The model under review builds one solid part; all positions refer to its coordinate system, in mm. Coordinates: 2 decimals unless noted, no trailing zeros. Loops run counter-clockwise (first coordinate to the right, second up) from the corner with the lowest first, then second, coordinate; pieces in that order, holes last. Notation, with made-up numbers: (-30, 83) - (27, 83) arc R15 ccw to (27, 97) - close; hole circle Ø8 at (-5.75, 38). An arc over 180 degrees is marked (long way). Answer in a Markdown table with one row per item. Add a question column.
(1) For P1, Ø5.5, axis at x = 137.85, z = -83.65, coming from the +Y side; P2, Ø2.5, axis at x = -47.65, z = 80.65, coming from the -Y side; P3, Ø1.5, axis at x = -39, y = 7, coming from the +Z side (3 decimals); P4, Ø5, axis at x = 54.5, z = 102, coming from the +Y side, all flat-tipped, find the tip position at first contact; note any pin that passes through.
(2) We need section B-B on x = 194. Write out the cut boundary in (y, z) (3 decimals), plus the area to 3 significant figures.
(3) For line 1 along X through (y, z) = (5, -0.5); line 2 along Z through (x, y) = (-159, 7.5) (3 decimals); line 3 along X through (y, z) = (7.25, 4), list the stretches that pass through material, from the lowest coordinate up.
(4) We need section A-A on y = 8. Give the number of separate pieces and of enclosed holes in the cut face, plus the area to 3 significant figures.
from build123d import *

# Parameters (mm, degrees)
SKETCH3_W           = 469.9
SKETCH3_H           = 209.55
BOSS_EXTRUDE1_DEPTH = 10
SKETCH4_R           = 2.1
CUT_EXTRUDE3_DEPTH  = 258.447670654
SKETCH5_R           = 2.1
CUT_EXTRUDE4_DEPTH  = 258.447670654
SKETCH7_W           = 25.4
SKETCH7_H           = 25.4
CUT_EXTRUDE5_DEPTH  = 6.35
CUT_EXTRUDE6_REACH  = 483.543
SKETCH8_W           = 6.35
SKETCH8_H           = 5.08
FILLET1_R           = 6.35


with BuildPart() as part:
    # Sketch3 → Boss-Extrude1 (new body)
    with BuildSketch(Plane(origin=(0, 0, 0), x_dir=(1, 0, 0), z_dir=(0, 1, 0))):
        Rectangle(SKETCH3_W, SKETCH3_H)
    extrude(amount=BOSS_EXTRUDE1_DEPTH)

    # Sketch4 → Cut-Extrude3 (cut, through all)
    with BuildSketch(Plane(origin=(0, 10, 0), x_dir=(1, 0, 0), z_dir=(0, 1, 0))):
        with Locations(Location((-102.9, 83.65, 0), (0, 0, 270))):
            Circle(SKETCH4_R)
        with Locations(Location((-22.65, 83.65, 0), (0, 0, 270))):
            Circle(SKETCH4_R)
        with Locations(Location((57.6, 83.65, 0), (0, 0, 270))):
            Circle(SKETCH4_R)
        with Locations(Location((137.85, 83.65, 0), (0, 0, 270))):
            Circle(SKETCH4_R)
        with Locations(Location((112.85, -80.65, 0), (0, 0, 270))):
            Circle(SKETCH4_R)
        with Locations(Location((32.6, -80.65, 0), (0, 0, 270))):
            Circle(SKETCH4_R)
        with Locations(Location((-47.65, -80.65, 0), (0, 0, 270))):
            Circle(SKETCH4_R)
        with Locations(Location((-127.9, -80.65, 0), (0, 0, 270))):
            Circle(SKETCH4_R)
    extrude(amount=-CUT_EXTRUDE3_DEPTH, mode=Mode.SUBTRACT)

    # Sketch5 → Cut-Extrude4 (cut, through all)
    with BuildSketch(Plane(origin=(0, 10, 0), x_dir=(1, 0, 0), z_dir=(0, 1, 0))):
        with Locations(Location((-137.85, 83.65, 0), (0, 0, 270))):
            Circle(SKETCH5_R)
        with Locations(Location((-57.6, 83.65, 0), (0, 0, 270))):
            Circle(SKETCH5_R)
        with Locations(Location((22.65, 83.65, 0), (0, 0, 270))):
            Circle(SKETCH5_R)
        with Locations(Location((102.9, 83.65, 0), (0, 0, 270))):
            Circle(SKETCH5_R)
        with Locations(Location((-112.85, -80.65, 0), (0, 0, 270))):
            Circle(SKETCH5_R)
        with Locations(Location((-32.6, -80.65, 0), (0, 0, 270))):
            Circle(SKETCH5_R)
        with Locations(Location((47.65, -80.65, 0), (0, 0, 270))):
            Circle(SKETCH5_R)
        with Locations(Location((127.9, -80.65, 0), (0, 0, 270))):
            Circle(SKETCH5_R)
    extrude(amount=-CUT_EXTRUDE4_DEPTH, mode=Mode.SUBTRACT)

    # Sketch7 → Cut-Extrude5 (cut)
    with BuildSketch(Plane(origin=(0, 10, 0), x_dir=(1, 0, 0), z_dir=(0, 1, 0))):
        with Locations((-180.25, 3.175)):
            Rectangle(SKETCH7_W, SKETCH7_H)
    extrude(amount=-CUT_EXTRUDE5_DEPTH, mode=Mode.SUBTRACT)

    # Sketch8 → Cut-Extrude6 (cut, up to next)
    with BuildSketch(Plane.ZY.offset(234.95), mode=Mode.PRIVATE) as cut_extrude6_sk1:
        with Locations((101.6, 7.46)):
            Rectangle(SKETCH8_W, SKETCH8_H)
    cut_extrude6_tool1 = extrude(cut_extrude6_sk1.sketch, amount=-CUT_EXTRUDE6_REACH, mode=Mode.PRIVATE) & part.part
    add(cut_extrude6_tool1.solids().sort_by_distance((-234.95, 7.46, 101.6))[0], mode=Mode.SUBTRACT)

    # Fillet1
    fillet1_edges = [part.edges().sort_by_distance(p)[0] for p in [
        (-167.55, 6.825, -15.875),
        (-167.55, 6.825, 9.525),
        (-192.95, 6.825, 9.525),
        (-192.95, 6.825, -15.875),
    ]]
    fillet(fillet1_edges, radius=FILLET1_R)


solid = part.part
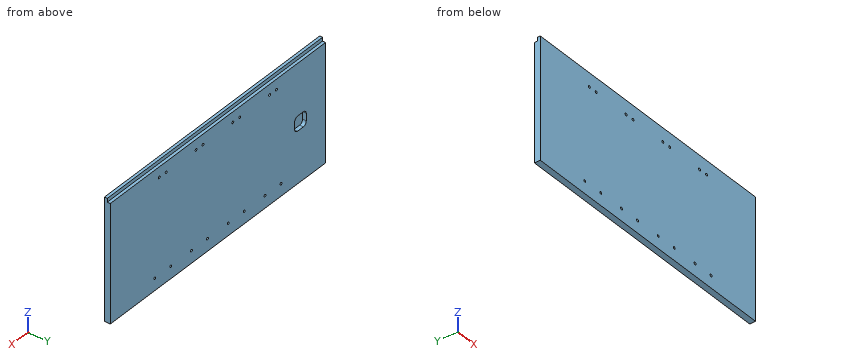
Outcome:
| question | item | result |
|---|---|---|
| 1 | P1 | y = 10 |
| 1 | P2 | through |
| 1 | P3 | z = 98.425 |
| 1 | P4 | y = 4.92 |
| 2 | outline | (0, -104.775) - (10, -104.775) - (10, 98.425) - (4.92, 98.425) - (4.92, 104.775) - (0, 104.775) - close |
| 2 | area | 2,060 mm² |
| 3 | line 1 | -234.95 to -192.95, -167.55 to 234.95 |
| 3 | line 2 | -104.775 to 98.425 |
| 3 | line 3 | -234.95 to -192.9, -167.6 to 234.95 |
| 4 | separate pieces | 1 |
| 4 | enclosed holes | 17 |
| 4 | area | 94,700 mm² |
